Here's how the part is built. I have some questions about the finished solid (model axes, mm). Give positions to 0.01 mm unless a question says otherwise; leave off trailing zeros. Loops run counter-clockwise (first coordinate to the right, second up) from the corner with the lowest first, then second, coordinate; pieces in that order, holes last. Notation, with made-up numbers: (31, -28.75) -> (78, -28.75) arc R35 cw to (78, 6.25) -> close; hole circle Ø2 at (66, 31). An arc over 180 degrees is marked (long way). Answer in a Markdown table with one row per item. Add a question column.
Item 1: For P1, Ø3, axis at x = 2, y = 140.5, coming from the -Z side; P2, Ø1.7, axis at y = 140.5, z = -56.5, coming from the -X side; P3, Ø3, axis at x = 2.5, y = 139.5, coming from the +Z side, each with a flat end and sliding along its axis, tell me the tip position at first contact or that it passes through.
Item 2: If we section it at A-A (z = -81.5): Write out the boundary of the cut face in (x, y) (3 decimals), then the cut area to 3 significant figures.
Item 3: If I drill on line 1 (X direction, y = 141.85, z = 22.5), over which ranges is the centre line in solid material (lowest first)?
```python
from build123d import *

# Parameters (mm, degrees)
SKETCH1_W           = 279.4
SKETCH1_H           = 285.75
BOSS_EXTRUDE1_DEPTH = 5.588
SKETCH2_W           = 279.4
SKETCH2_H           = 5.588
BOSS_EXTRUDE2_DEPTH = 12.7
CUT_EXTRUDE1_DEPTH  = 19.288
SKETCH5_W           = 64.162912319
SKETCH5_H           = 368.728813298
CUT_EXTRUDE2_DEPTH  = 280.4
SKETCH4_W           = 12.7
SKETCH4_H           = 5.588
CUT_EXTRUDE3_DEPTH  = 6.35


with BuildPart() as part:
    # Sketch1 → Boss-Extrude1 (new body)
    with BuildSketch(Plane(origin=(0, 0, 0), x_dir=(0, 0, -1), z_dir=(1, 0, 0))):
        Rectangle(SKETCH1_W, SKETCH1_H)
    extrude(amount=BOSS_EXTRUDE1_DEPTH)

    # Sketch2 → Boss-Extrude2 (add)
    with BuildSketch(Plane(origin=(5.588, 0, 0), x_dir=(0, 0, -1), z_dir=(1, 0, 0))):
        with Locations((0, 140.081)):
            Rectangle(SKETCH2_W, SKETCH2_H)
    extrude(amount=BOSS_EXTRUDE2_DEPTH)

    # Sketch3 → Cut-Extrude1 (cut, through all)
    with BuildSketch(Plane.ZY):
        with BuildLine():
            Line((-114.3, -85.725), (-25.4, -85.725))
            ThreePointArc((-25.4, -85.725), (-12.7, -98.425), (-25.4, -111.125))
            Line((-25.4, -111.125), (-114.3, -111.125))
            ThreePointArc((-114.3, -111.125), (-127, -98.425), (-114.3, -85.725))
        make_face()
    extrude(amount=-CUT_EXTRUDE1_DEPTH, mode=Mode.SUBTRACT)

    # Sketch5 → Cut-Extrude2 (cut, through all)
    with BuildSketch(Plane(origin=(0, 0, -139.7), x_dir=(-1, 0, 0), z_dir=(0, 0, -1))):
        with Locations((13.79345616, -47.077406649)):
            Rectangle(SKETCH5_W, SKETCH5_H)
    extrude(amount=-CUT_EXTRUDE2_DEPTH, mode=Mode.SUBTRACT)

    # Sketch4 → Cut-Extrude3 (cut)
    with BuildSketch(Plane.ZY):
        with Locations((-106.68, 140.081)):
            Rectangle(SKETCH4_W, SKETCH4_H)
        with Locations((-133.35, 140.081)):
            Rectangle(SKETCH4_W, SKETCH4_H)
        with Locations((-80.01, 140.081)):
            Rectangle(SKETCH4_W, SKETCH4_H)
        with Locations((-53.34, 140.081)):
            Rectangle(SKETCH4_W, SKETCH4_H)
        with Locations((-26.67, 140.081)):
            Rectangle(SKETCH4_W, SKETCH4_H)
        with Locations((0, 140.081)):
            Rectangle(SKETCH4_W, SKETCH4_H)
        with Locations((26.67, 140.081)):
            Rectangle(SKETCH4_W, SKETCH4_H)
        with Locations((53.34, 140.081)):
            Rectangle(SKETCH4_W, SKETCH4_H)
        with Locations((80.01, 140.081)):
            Rectangle(SKETCH4_W, SKETCH4_H)
        with Locations((106.68, 140.081)):
            Rectangle(SKETCH4_W, SKETCH4_H)
        with Locations((133.35, 140.081)):
            Rectangle(SKETCH4_W, SKETCH4_H)
    extrude(amount=-CUT_EXTRUDE3_DEPTH, mode=Mode.SUBTRACT)


solid = part.part
```
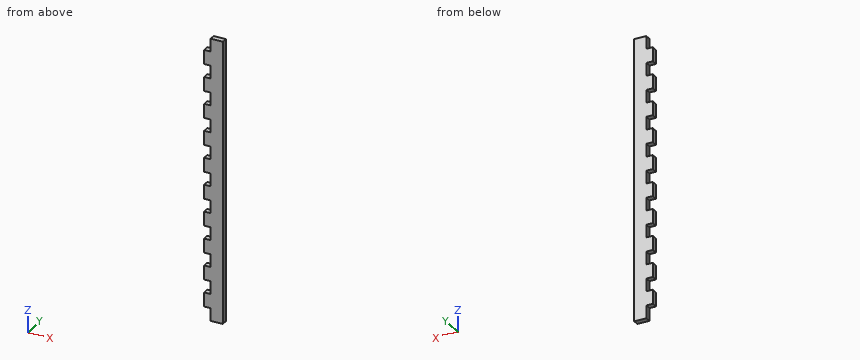
Recorded:
| question | item | result |
|---|---|---|
| 1 | P1 | stops at z = -127 |
| 1 | P2 | stops at x = 6.35 |
| 1 | P3 | stops at z = 127 |
| 2 | outline | (6.35, 137.287) -> (18.288, 137.287) -> (18.288, 142.875) -> (6.35, 142.875) -> close |
| 2 | area | 66.7 mm^2 |
| 3 | line 1 | x = 6.35 to 18.29 |
